Part model, mm, in its own coordinate system. A direction names the side the tool comes from. Coordinates: 2 decimals unless noted, no trailing zeros. Order: outer loops, then holes, each group sorted by start corner. A loop starts at its lowest first (then second) coordinate and runs counter-clockwise, first axis right, second up.
from build123d import *

# Parameters (mm, degrees)
F0_W     = 286
F0_H     = 180
F1_DEPTH = 6.2
F2_W     = 12
F2_H     = 6.2
F2_W_2   = 5
F3_DEPTH = 6.201
F4_W     = 286
F4_H     = 61.5
F5_DEPTH = 6.201
F6_W     = 6.2
F6_H     = 12
F6_H_2   = 10.5
F7_DEPTH = 6.2


with BuildPart() as f1:
    # F0 (on Front) → F1 (new body)
    with BuildSketch(Plane.XZ):
        Rectangle(F0_W, F0_H)
    extrude(amount=F1_DEPTH)

    # F2 (on face) → F3 (cut, through all)
    with BuildSketch(Plane.XZ.offset(6.2)):
        with Locations((-120, -25.4)):
            Rectangle(F2_W, F2_H)
        with Locations((-96, -25.4)):
            Rectangle(F2_W, F2_H)
        with Locations((-72, -25.4)):
            Rectangle(F2_W, F2_H)
        with Locations((-48, -25.4)):
            Rectangle(F2_W, F2_H)
        with Locations((-24, -25.4)):
            Rectangle(F2_W, F2_H)
        with Locations((0, -25.4)):
            Rectangle(F2_W, F2_H)
        with Locations((24, -25.4)):
            Rectangle(F2_W, F2_H)
        with Locations((48, -25.4)):
            Rectangle(F2_W, F2_H)
        with Locations((72, -25.4)):
            Rectangle(F2_W, F2_H)
        with Locations((96, -25.4)):
            Rectangle(F2_W, F2_H)
        with Locations((120, -25.4)):
            Rectangle(F2_W, F2_H)
        with Locations((-140.5, -25.4)):
            Rectangle(F2_W_2, F2_H)
        with Locations((140.5, -25.4)):
            Rectangle(F2_W_2, F2_H)
    extrude(amount=-F3_DEPTH, mode=Mode.SUBTRACT)

    # F4 (on face) → F5 (cut, through all)
    with BuildSketch(Plane.XZ.offset(6.2)):
        with Locations((0, -59.25)):
            Rectangle(F4_W, F4_H)
    extrude(amount=-F5_DEPTH, mode=Mode.SUBTRACT)

    # F6 (on face) → F7 (join)
    with BuildSketch(Plane.XZ.offset(6.2)):
        with Locations((-146.1, 72)):
            Rectangle(F6_W, F6_H)
        with Locations((-146.1, 48)):
            Rectangle(F6_W, F6_H)
        with Locations((-146.1, 24)):
            Rectangle(F6_W, F6_H)
        with Locations((-146.1, 0)):
            Rectangle(F6_W, F6_H)
        with Locations((-146.1, -23.25)):
            Rectangle(F6_W, F6_H_2)
        with Locations((146.1, 48)):
            Rectangle(F6_W, F6_H)
        with Locations((146.1, 72)):
            Rectangle(F6_W, F6_H)
        with Locations((146.1, 24)):
            Rectangle(F6_W, F6_H)
        with Locations((146.1, 0)):
            Rectangle(F6_W, F6_H)
        with Locations((146.1, -23.25)):
            Rectangle(F6_W, F6_H_2)
    extrude(amount=-F7_DEPTH)


solid = f1.part
Q1. Cut at B-B on x = -1.5. Write the cut outline in (y, z).
Results list:
outline: (-6.2, -22.3) - (0, -22.3) - (0, 90) - (-6.2, 90) - close
Q2. Cut at A-A on z = 39. Write the cut outline in (x, y).
Results list:
outline: (-143, -6.2) - (143, -6.2) - (143, 0) - (-143, 0) - close
Q3. Wall check: line 1 along Z through (x, y) = (91, -2); line 2 along X through (y, z) = (-3.25, 62). Give the ranges that are in metal, low to high.
Results list:
line 1: z = -22.3 to 90
line 2: x = -143 to 143
Q4. Pin check, flat tips, straight feed: pin 1 Ø1.9 at (x, y) = (147, -4.5) entering from +Z; pin 2 Ø3 at (y, z) = (-2, 13) entering from -X. Stop position of each tip, or through.
Results list:
pin 1: stops at z = 78
pin 2: stops at x = -143
Q5. Mould opens along X. For faces 5 (the face through (-149.2, -3, 48)), 6 (the face through (143, -3, 84)), 7 (the face through (-48, -3, -22.3)) say: pulls with the +X half, pulls with the -X half, needs draft (parallel to the pull), parting line crosses it, or undercut.
Results list:
face 5: pulls with the -X half
face 6: pulls with the +X half
face 7: undercut
Q6. Which spindle directions (+Z, -Z, +X, -X, +Y, -Y) get a long thin tool onto all of the face, cutting with end or side? Do faces 1 (the face through (-114, -3, -25)), 2 (the face through (146, -3, 42)), 3 (the face through (146, -3, 78)), 4 (the face through (-146, -3, 18)). Say none if no direction does.
Results list:
face 1: -Z, +Y, -Y
face 2: +X, +Y, -Y
face 3: +Z, +X, +Y, -Y
face 4: -X, +Y, -Y
